The drawing under review shows one solid part. Ordinate dimensions are in mm from its lowest x, y, z. Give positions to 0.01 mm unless a question says otherwise; leave off trailing zeros. Loops run counter-clockwise (first coordinate to the right, second up) from the corner with the lowest first, then second, coordinate; pieces in that order, holes last. Notation, with made-up numbers: (88.25, 11.25) - (104.25, 11.25) arc R30 ccw to (104.25, 42.25) - close; hole circle Ø9 at (-13, 10). An arc over 180 degrees is marked (long way). Write each question's results on one line, items separated by ' | '.
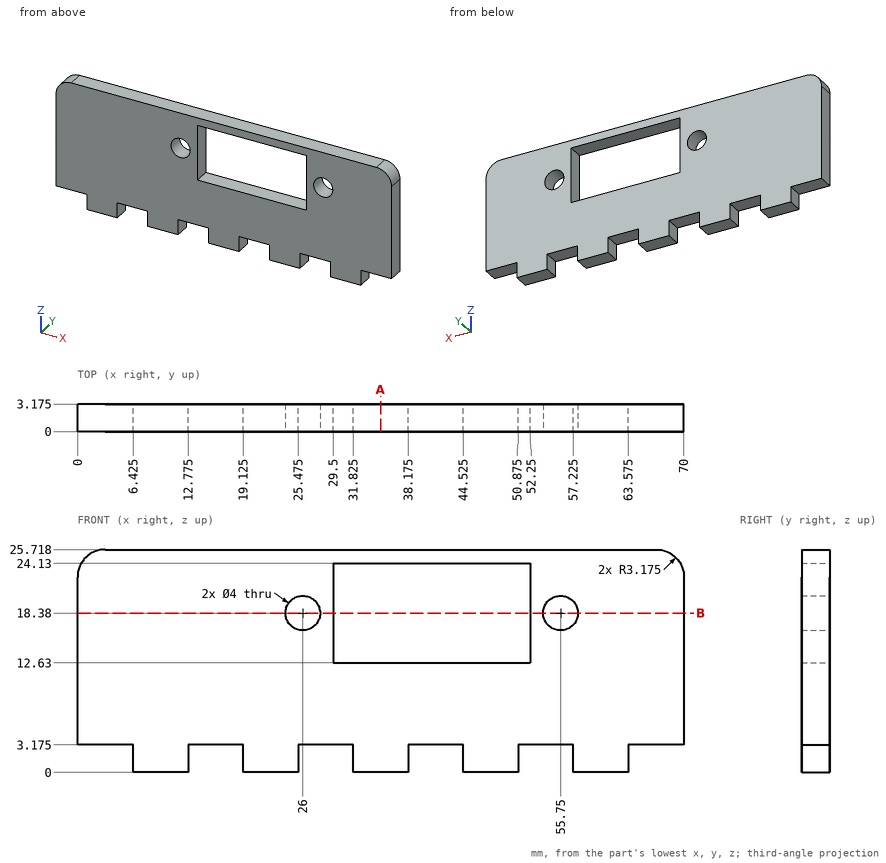
(1) Insertion check: P1, Ø1.6, axis at y = 1.5, z = 1.5, coming from the -X side (1 decimal); P2, Ø1, axis at x = 42.5, y = 2, coming from the -Z side (1 decimal); P3, Ø1.6, axis at y = 1, z = 1.5, coming from the +X side (1 decimal). Each pin has a flat end and moves straight along its axis. Give the tip position at first contact, or say it passes through.
Answers below:
P1: x = 6.4 | P2: z = 3.2 | P3: x = 63.6
(2) Take a section at B-B on z = 18.38. Count the separate pieces of the cut face and the enclosed holes in it, plus the area to 3 significant figures.
Answers below:
separate pieces: 4 | enclosed holes: 0 | area: 125 mm2
(3) Wall thickness on line 1 along X through (y, z) = (3, 1.5) (1 decimal); line 2 along X through (y, z) = (1.3, 18.38); line 3 along Z through (x, y) = (51, 0.35) (1 decimal): over which ranges is each line inside the solid? List them lowest first. Write a range as from..to.
Answers below:
line 1: 6.4..12.8, 19.1..25.5, 31.8..38.2, 44.5..50.9, 57.2..63.6 | line 2: 0..24, 28..29.5, 52.25..53.75, 57.75..70 | line 3: 3.2..12.6, 24.1..25.7
(4) Take a section at A-A on x = 35. Give the boundary of the cut face in (y, z) (1 decimal).
Answers below:
outline: (0, 0) - (3.2, 0) - (3.2, 12.6) - (0, 12.6) - close; (0, 24.1) - (3.2, 24.1) - (3.2, 25.7) - (0, 25.7) - close
